from build123d import *

# Parameters (mm, degrees)
SKETCH_1_R      = 4
SKETCH_1_R_2    = 3
EXTRUDE_1_DEPTH = 0.7
SKETCH_2_R      = 7
SKETCH_2_R_2    = 3
EXTRUDE_2_DEPTH = 0.7


with BuildPart() as part:
    # 草图1 → 凸台-拉伸1 (new body)
    with BuildSketch(Plane.XY):
        Circle(SKETCH_1_R)
        Circle(SKETCH_1_R_2, mode=Mode.SUBTRACT)
    extrude(amount=-EXTRUDE_1_DEPTH)

    # 草图2 → 凸台-拉伸2 (add)
    with BuildSketch(Plane(origin=(0, 0, -0.7), x_dir=(-1, 0, 0), z_dir=(0, 0, -1))):
        Circle(SKETCH_2_R)
        with Locations(Location((0, 0, 0), (0, 0, 180))):
            Circle(SKETCH_2_R_2, mode=Mode.SUBTRACT)
    extrude(amount=EXTRUDE_2_DEPTH)


solid = part.part
Can you work these out from the model? Positions are in its coordinate system, mm. A direction names the side the tool comes from. Give positions to 0.01 mm unless a question says otherwise; leave off trailing zeros. Loops run counter-clockwise (first coordinate to the right, second up) from the corner with the lowest first, then second, coordinate; pieces in that order, holes last. Notation, with made-up numbers: M 63.25,66.5 L 118.25,66.5 A20 cw 118.25,102.5 Z; hole C 11.5,79 d10. An arc over 180 degrees is marked long. One line per item, written item: value. Start each with the question number.
1) If we section it at C-C, the plane z = -1.05: Write out the boundary of the cut face in (x, y).
2) If we section it at D-D, the plane y = 5.5: Write out the boundary of the cut face in (x, z).
3) If I drill on line 1 (Y direction, x = 0, z = -0.5); line 2 (Y direction, x = 0, z = -1.2); line 3 (Z direction, x = -5, y = 4.5), over which ranges is the centre line in solid material (lowest first)? Write a range as [from, to].
4) If we section it at A-A, the plane x = 0: Write out the boundary of the cut face in (y, z), and give its area (3 significant figures).
5) On a 3-axis mill with a long thin cutter (end or side, diameter ignored), from which of +Z, -Z, +X, -X, +Y, -Y can I reach the whole of each face in a straight line? I mean faces 1 (the face through (-6.466, -2.681, -1.045)), 2 (the face through (-0.867, -3.905, -0.345)). Say none if no direction works.
Completed:
1. outline: C 0,0 d14; hole C 0,0 d6
2. outline: M -4.33,-1.4 L 4.33,-1.4 L 4.33,-0.7 L -4.33,-0.7 Z
3. line 1: y = [-4, -3], [3, 4]
3. line 2: y = [-7, -3], [3, 7]
3. line 3: z = [-1.4, -0.7]
4. outline: M -7,-1.4 L -3,-1.4 L -3,0 L -4,0 L -4,-0.7 L -7,-0.7 Z; M 3,-1.4 L 7,-1.4 L 7,-0.7 L 4,-0.7 L 4,0 L 3,0 Z
4. area: 7.00 mm^2
5. face 1: +Z, -Z
5. face 2: +Z
